Can you work these out from the model? Positions are in its coordinate system, mm. Coordinates: 2 decimals unless noted, no trailing zeros. Loops run counter-clockwise (first coordinate to the right, second up) from the corner with the lowest first, then second, coordinate; pieces in that order, holes last.
```python
from build123d import *

# Parameters (mm, degrees)
SKETCH1_R          = 7.5
BOSS_EXTRUDE_DEPTH = 50.8
DRAFT3_ANGLE       = 5
SKETCH2_R          = 4.5
CUT_EXTRUDE1_DEPTH = 54.534834776


with BuildPart() as part:
    # Sketch1 → Boss-Extrude (new body)
    with BuildSketch(Plane.XY):
        Circle(SKETCH1_R)
    extrude(amount=BOSS_EXTRUDE_DEPTH)

    # Draft3
    draft3_faces = [part.faces().sort_by_distance(p)[0] for p in [
        (-7.5, 0, 25.4),
    ]]
    draft(draft3_faces, Plane.XY.offset(50.8), DRAFT3_ANGLE)

    # Sketch2 → Cut-Extrude1 (cut, through all)
    with BuildSketch(Plane(origin=(0, 0, 0), x_dir=(-1, 0, 0), z_dir=(0, 0, -1))):
        Circle(SKETCH2_R)
    extrude(amount=-CUT_EXTRUDE1_DEPTH, mode=Mode.SUBTRACT)


solid = part.part
```
Item 1: I need wall thicknesses on line 1 along Y through (x, z) = (0, 36.5); line 2 along Y through (x, z) = (0, 16); line 3 along X through (y, z) = (-1.25, 30). Which ranges of each line are inside material? Lowest first, please.
Results are:
line 1: y = -8.75 to -4.5, 4.5 to 8.75
line 2: y = -10.54 to -4.5, 4.5 to 10.54
line 3: x = -9.24 to -4.32, 4.32 to 9.24
Item 2: We'd pull the mould along X, two halves only. Please class faces 1 (the face through (0, -5, 50.8)), 2 (the face through (0.59, 4.46, 25.04)), 3 (the face through (-2.114, -9.521, 25.044)): +X half, -X half, draft (parallel to the pull), parting line (faces both ways), or undercut.
Results are:
face 1: draft
face 2: undercut
face 3: parting line
Item 3: I'm going to push flat-ended pins straight in: P1, Ø5, axis at x = -0.5, z = 45.5, coming from the -Y side; P2, Ø1, axis at x = -1.5, z = 37.5, coming from the +Y side; P3, Ø2, axis at y = 0, z = 26, coming from the -X side. Where does each tip first touch, or does it pass through?
Results are:
P1: stops at y = -8.18
P2: stops at y = 8.62
P3: stops at x = -9.76
Item 4: Suppose I cut it at A-A, the plane y = 0. Please give me the cut outline in (x, z).
Results are:
outline: (-11.94, 0) - (-4.5, 0) - (-4.5, 50.8) - (-7.5, 50.8) - close; (4.5, 0) - (11.94, 0) - (7.5, 50.8) - (4.5, 50.8) - close
Item 5: Suppose I cut it at D-D, the plane z = 9.5. Please give me the cut outline in (x, y), plus the area to 3 significant figures.
Results are:
outline: circle Ø22.23 at (0, 0); hole circle Ø9 at (0, 0)
area: 324 mm2
Item 6: Suppose I cut it at C-C, the plane z = 27. Please give me the cut outline in (x, y), plus the area to 3 significant figures.
Results are:
outline: circle Ø19.16 at (0, 0); hole circle Ø9 at (0, 0)
area: 225 mm2
